from build123d import *

# Parameters (mm, degrees)
SKETCH1_W                 = 457.223
SKETCH1_H                 = 367.60800004
BOSS_EXTRUDE2_DEPTH       = 3.175
SKETCH4_W                 = 3.175
SKETCH4_H                 = 80
CUT_EXTRUDE1_DEPTH        = 3.175
LPATTERN1_COUNT           = 4
LPATTERN1_PITCH           = 90.807
LPATTERN1_COPY_1_SKETCH_W = 3.175
LPATTERN1_COPY_1_SKETCH_H = 80
LPATTERN1_COPY_1_DEPTH    = 3.175
LPATTERN1_COPY_2_SKETCH_W = 3.175
LPATTERN1_COPY_2_SKETCH_H = 80
LPATTERN1_COPY_2_DEPTH    = 3.175
LPATTERN1_COPY_3_SKETCH_W = 3.175
LPATTERN1_COPY_3_SKETCH_H = 80
LPATTERN1_COPY_3_DEPTH    = 3.175
SKETCH5_W                 = 49.658811606
SKETCH5_H                 = 3.175
CUT_EXTRUDE2_DEPTH        = 3.175
MIRROR3_COPY_1_SKETCH_W   = 49.658811606
MIRROR3_COPY_1_SKETCH_H   = 3.175
MIRROR3_COPY_1_DEPTH      = 3.175
SKETCH6_W                 = 3.175
SKETCH6_H                 = 80
CUT_EXTRUDE3_DEPTH        = 311.705796904
SKETCH8_W                 = 44.275
SKETCH8_H                 = 95.25
SKETCH8_W_2               = 93.98
SKETCH8_H_2               = 44.45
BOSS_EXTRUDE3_DEPTH       = 3.175
M6_CLEARANCE_HOLE1_D      = 7


with BuildPart() as part:
    # Sketch1 → Boss-Extrude2 (new body)
    with BuildSketch(Plane.XY):
        with Locations((0, -26.588)):
            Rectangle(SKETCH1_W, SKETCH1_H)
    extrude(amount=BOSS_EXTRUDE2_DEPTH)

    # Sketch4 → Cut-Extrude1 (cut)
    with BuildSketch(Plane.XY.offset(3.175)):
        with Locations((-136.213, 77.21600002)):
            Rectangle(SKETCH4_W, SKETCH4_H)
    cut_extrude1 = extrude(amount=-CUT_EXTRUDE1_DEPTH, mode=Mode.SUBTRACT)

    # Mirror1: Cut-Extrude1 across plane
    add(cut_extrude1.mirror(Plane.ZX), mode=Mode.SUBTRACT)

    # LPattern1: Cut-Extrude1 ×4
    with Locations(*[(i * LPATTERN1_PITCH, 0, 0) for i in range(1, LPATTERN1_COUNT)]):
        add(cut_extrude1, mode=Mode.SUBTRACT)

    # LPattern1 copy 1 sketch → LPattern1 copy 1 (cut)
    with BuildSketch(Plane(origin=(90.807, 0, 3.175), x_dir=(1, 0, 0), z_dir=(0, 0, 1))):
        with Locations((-136.213, -77.21600002)):
            Rectangle(LPATTERN1_COPY_1_SKETCH_W, LPATTERN1_COPY_1_SKETCH_H)
    extrude(amount=-LPATTERN1_COPY_1_DEPTH, mode=Mode.SUBTRACT)

    # LPattern1 copy 2 sketch → LPattern1 copy 2 (cut)
    with BuildSketch(Plane(origin=(181.614, 0, 3.175), x_dir=(1, 0, 0), z_dir=(0, 0, 1))):
        with Locations((-136.213, -77.21600002)):
            Rectangle(LPATTERN1_COPY_2_SKETCH_W, LPATTERN1_COPY_2_SKETCH_H)
    extrude(amount=-LPATTERN1_COPY_2_DEPTH, mode=Mode.SUBTRACT)

    # LPattern1 copy 3 sketch → LPattern1 copy 3 (cut)
    with BuildSketch(Plane(origin=(272.421, 0, 3.175), x_dir=(1, 0, 0), z_dir=(0, 0, 1))):
        with Locations((-136.213, -77.21600002)):
            Rectangle(LPATTERN1_COPY_3_SKETCH_W, LPATTERN1_COPY_3_SKETCH_H)
    extrude(amount=-LPATTERN1_COPY_3_DEPTH, mode=Mode.SUBTRACT)

    # Sketch5 → Cut-Extrude2 (cut)
    with BuildSketch(Plane.XY.offset(3.175)):
        with Locations((-91.020094169, -155.62850002)):
            Rectangle(SKETCH5_W, SKETCH5_H)
    cut_extrude2 = extrude(amount=-CUT_EXTRUDE2_DEPTH, mode=Mode.SUBTRACT)

    # Mirror2: Cut-Extrude2 across plane
    add(cut_extrude2.mirror(Plane(origin=(0, 0, 0), x_dir=(0, 0, 1), z_dir=(1, 0, 0))), mode=Mode.SUBTRACT)

    # Mirror3: Cut-Extrude2 across plane
    add(cut_extrude2.mirror(Plane.ZX), mode=Mode.SUBTRACT)

    # Mirror3 copy 1 sketch → Mirror3 copy 1 (cut)
    with BuildSketch(Plane(origin=(0, 0, 3.175), x_dir=(-1, 0, 0), z_dir=(0, 0, 1))):
        with Locations((-91.020094169, -155.62850002)):
            Rectangle(MIRROR3_COPY_1_SKETCH_W, MIRROR3_COPY_1_SKETCH_H)
    extrude(amount=-MIRROR3_COPY_1_DEPTH, mode=Mode.SUBTRACT)

    # Sketch6 → Cut-Extrude3 (cut, through all)
    with BuildSketch(Plane.XY.offset(3.175)):
        with Locations((-227.024, -2.78399998)):
            Rectangle(SKETCH6_W, SKETCH6_H)
    cut_extrude3 = extrude(amount=-CUT_EXTRUDE3_DEPTH, mode=Mode.SUBTRACT)

    # Mirror5: Cut-Extrude3 across plane
    add(cut_extrude3.mirror(Plane(origin=(0, 0, 0), x_dir=(0, 0, 1), z_dir=(1, 0, 0))), mode=Mode.SUBTRACT)

    # Sketch8 → Boss-Extrude3 (add)
    with BuildSketch(Plane(origin=(0, 0, 0), x_dir=(-1, 0, 0), z_dir=(0, 0, -1))):
        with Locations((-250.749, 109.59100002)):
            Rectangle(SKETCH8_W, SKETCH8_H)
        with Locations((-181.6215, 179.44100002)):
            Rectangle(SKETCH8_W_2, SKETCH8_H_2)
        with Locations((-250.749, -109.59100002)):
            Rectangle(SKETCH8_W, SKETCH8_H)
    boss_extrude3 = extrude(amount=-BOSS_EXTRUDE3_DEPTH)

    # Mirror7: Boss-Extrude3 across plane
    add(boss_extrude3.mirror(Plane(origin=(0, 0, 0), x_dir=(0, 0, 1), z_dir=(1, 0, 0))))

    # M6 Clearance Hole1 (through all)
    with Locations(Plane(origin=(0, 0, 0), x_dir=(-1, 0, 0), z_dir=(0, 0, -1))):
        with Locations((-254.0115, -135.59100002), (-254.0115, -83.59100002), (-254.0115, 83.59100002), (-254.0115, 135.59100002), (-181.6215, 179.44100002)):
            m6_clearance_hole1 = Hole(M6_CLEARANCE_HOLE1_D / 2)

    # Mirror8: M6 Clearance Hole1 across plane
    add(m6_clearance_hole1.mirror(Plane(origin=(0, 0, 0), x_dir=(0, 0, 1), z_dir=(1, 0, 0))), mode=Mode.SUBTRACT)


solid = part.part
Read the model definition and answer for the solid it produces. Units are mm, in the model's axes. Round coordinates to 2 decimals unless told otherwise and drop trailing zeros. Order: outer loops, then holes, each group sorted by start corner. A loop starts at its lowest first (then second) coordinate and runs counter-clockwise, first axis right, second up.
1) The part is cut by section C-C on y = 99. Write down the section's boundary in (x, z) (1 decimal), plus the area to 3 significant figures.
2) The part is cut by section D-D on x = 54.5. Write down the section's boundary in (y, z) (3 decimals), plus the area to 3 significant figures.
3) The part is cut by section B-B on x = -92. Write down the section's boundary in (y, z) (3 decimals), plus the area to 3 significant figures.
4) Straight lines are drawn through the part: L1, parallel to X at y = -111.5, z = 2.3; L2, parallel to X at y = 156.5, z = 0.75; L3, parallel to X at y = 55, z = 2.5. For each, find the intervals that lie inside material, in ascending order.
5) Flat-ended cylindrical pins translate along their axes: pin 1 (1 mm diameter, centred on x = -121.5, z = 1.5, fed in from +Y); pin 2 (1.6 mm diameter, centred on y = 13, z = 2, fed in from -X); pin 3 (11 mm diameter, centred on x = -254.01, y = -135.59, fed in from +Z) (3 decimals); pin 4 (1.6 mm diameter, centred on y = 53.5, z = 1.5, fed in from -X). Find the tip coordinate at first contact, or state that the pin passes through.
6) The part is cut by section A-A on y = 53.5. Write down the section's boundary in (x, z) (1 decimal), plus the area to 3 significant figures.
Resolved:
1. outline: (-272.9, 0) - (-137.8, 0) - (-137.8, 3.2) - (-272.9, 3.2) - close; (-134.6, 0) - (-47, 0) - (-47, 3.2) - (-134.6, 3.2) - close; (-43.8, 0) - (43.8, 0) - (43.8, 3.2) - (-43.8, 3.2) - close; (47, 0) - (134.6, 0) - (134.6, 3.2) - (47, 3.2) - close; (137.8, 0) - (272.9, 0) - (272.9, 3.2) - (137.8, 3.2) - close
1. area: 1,690 mm2
2. outline: (-210.392, 0) - (157.216, 0) - (157.216, 3.175) - (-210.392, 3.175) - close
2. area: 1,170 mm2
3. outline: (-210.392, 0) - (-157.216, 0) - (-157.216, 3.175) - (-210.392, 3.175) - close; (-154.041, 0) - (154.041, 0) - (154.041, 3.175) - (-154.041, 3.175) - close
3. area: 1,150 mm2
4. L1: x = -272.89 to -137.8, -134.63 to -46.99, -43.82 to 43.81, 46.99 to 134.62, 137.8 to 272.89
4. L2: x = -272.89 to -115.85, -66.19 to 66.19, 115.85 to 272.89
4. L3: x = -228.61 to -137.8, -134.63 to -46.99, -43.82 to 43.81, 46.99 to 134.62, 137.8 to 228.61
5. pin 1: stops at y = 157.22
5. pin 2: stops at x = -225.44
5. pin 3: stops at z = 3.175
5. pin 4: stops at x = -228.61
6. outline: (-228.6, 0) - (-137.8, 0) - (-137.8, 3.2) - (-228.6, 3.2) - close; (-134.6, 0) - (-47, 0) - (-47, 3.2) - (-134.6, 3.2) - close; (-43.8, 0) - (43.8, 0) - (43.8, 3.2) - (-43.8, 3.2) - close; (47, 0) - (134.6, 0) - (134.6, 3.2) - (47, 3.2) - close; (137.8, 0) - (228.6, 0) - (228.6, 3.2) - (137.8, 3.2) - close
6. area: 1,410 mm2
